from build123d import *

# Parameters (mm, degrees)
SKETCH1_W           = 13
SKETCH1_H           = 18
BOSS_EXTRUDE1_DEPTH = 3.2
SKETCH2_W           = 15
SKETCH2_H           = 20
BOSS_EXTRUDE2_DEPTH = 1
SKETCH3_R           = 1.5
CUT_EXTRUDE1_DEPTH  = 14.18673576
FILLET1_R           = 0.2
FILLET2_R           = 1


with BuildPart() as part:
    # Sketch1 → Boss-Extrude1 (new body)
    with BuildSketch(Plane(origin=(0, 0, 0), x_dir=(1, 0, 0), z_dir=(0, 1, 0))):
        Rectangle(SKETCH1_W, SKETCH1_H)
    extrude(amount=BOSS_EXTRUDE1_DEPTH)

    # Sketch2 → Boss-Extrude2 (add)
    with BuildSketch(Plane(origin=(0, 3.2, 0), x_dir=(1, 0, 0), z_dir=(0, 1, 0))):
        Rectangle(SKETCH2_W, SKETCH2_H)
    extrude(amount=BOSS_EXTRUDE2_DEPTH)

    # Sketch3 → Cut-Extrude1 (cut, through all)
    with BuildSketch(Plane.XZ):
        with Locations(Location((0, 3, 0), (0, 0, 270))):
            Circle(SKETCH3_R)
        with Locations(Location((0, -3, 0), (0, 0, 270))):
            Circle(SKETCH3_R)
        Polygon((4.8, -5.5), (-1.3, -5.5), (-1.3, -5.9), (5.5, -5.9), (5.5, 8), (4.8, 8), align=None)
        Polygon((2.5, 7.85), (2.5, -4.3), (3.6, -4.3), (3.6, 8), (-5.5, 8), (-5.5, 7.6), (1.5, 7.6), (1.5, 7.85), align=None)
        Polygon((-2.5, -7.1), (-2.5, 4.3), (-3.9, 4.3), (-3.9, -8), (5.5, -8), (5.5, -7.1), align=None)
        Polygon((-5.35, 5.5), (1.3, 5.5), (1.3, 6.4), (-5.5, 6.4), (-5.5, -8), (-5.1, -8), (-5.1, 4.3), (-5.35, 4.3), align=None)
    extrude(amount=-CUT_EXTRUDE1_DEPTH, mode=Mode.SUBTRACT)

    # Fillet1
    fillet1_edges = [part.edges().sort_by_distance(p)[0] for p in [
        (-5.1, 2.1, -8),
        (-3.9, 2.1, -8),
        (-5.5, 2.1, 6.4),
        (-5.5, 2.1, 7.6),
        (4.8, 2.1, 8),
        (3.6, 2.1, 8),
        (-3.9, 2.1, 4.3),
        (-2.5, 2.1, 4.3),
        (1.3, 2.1, 5.5),
        (1.3, 2.1, 6.4),
        (5.5, 2.1, -7.1),
        (5.5, 2.1, -5.9),
        (-1.3, 2.1, -5.9),
        (-1.3, 2.1, -5.5),
        (3.6, 2.1, -4.3),
        (2.5, 2.1, -4.3),
    ]]
    fillet(fillet1_edges, radius=FILLET1_R - 0.0001)  # a hair under: the kernel refuses the full size

    # Fillet2
    fillet2_edges = [part.edges().sort_by_distance(p)[0] for p in [
        (6.5, 1.6, 9),
        (-6.5, 1.6, 9),
        (-6.5, 1.6, -9),
        (6.5, 1.6, -9),
    ]]
    fillet(fillet2_edges, radius=FILLET2_R)


with BuildPart() as body_2:
    # Mirror1: mirrored copy
    add(part.part.mirror(Plane(origin=(-7.5, 4.2, -10), x_dir=(0, 0, 1), z_dir=(1, 0, 0))))


solid = body_2.part
CAD build for the part. Positions are in the model's coordinates, mm. A direction names the side the tool comes from. Give positions to 0.01 mm unless a question says otherwise; leave off trailing zeros. Loops run counter-clockwise (first coordinate to the right, second up) from the corner with the lowest first, then second, coordinate; pieces in that order, holes last. Notation, with made-up numbers: M -5,62.5 L -1,62.5 A13 cw -1,77.5 Z; hole C -30,-3 d5. An arc over 180 degrees is marked long. Answer in a Markdown table with one row per item. Add a question column.
Item 1: Mould opens along X. For faces 1 (the face through (-8.785, 1.622, 8.699)), 2 (the face through (-15, 4.2, 0)), 3 (the face through (-17, 2, 7.85)), 4 (the face through (-22.5, 4, 0)) say: +X half, -X half, draft (parallel to the pull), parting line (faces both ways), or undercut.
Item 2: Band-saw the part on A-A on z = 3. Give the cut face in (x, y), then the cut area to 3 significant figures.
Item 3: Tool access for faces 5 (the face through (-15, 2, -9)), 6 (the face through (-17, 2, -5.5)), 7 (the face through (-8.5, 2, 0)): list every direction of +Z, -Z, +X, -X, +Y, -Y with a clear straight run to the whole face (end or side of a thin tool).
Item 4: Drop flat-ended pins along their axis: P1, Ø1.3, axis at y = 2, z = 0.5, coming from the +X side; P2, Ø1.3, axis at y = 1.5, z = -3, coming from the -X side; P3, Ø2.5, axis at y = 2, z = 2.5, coming from the -X side; P4, Ø2, axis at x = -14, y = 2, coming from the +Z side. Give the stop position or say it passes through.
Item 5: Band-saw the part on B-B on x = -15. Give the number of separate pieces and of enclosed holes in the cut face, then the cut area to 3 significant figures.
Item 6: Probe probe 1 along Z at (x, y) = (-10.5, 1.7); probe 2 along Z at (x, y) = (-19.5, 1.45); probe 3 along X at (y, z) = (2.5, 5.75). List the from-to ranges inside material, lowest first.
Item 7: Band-saw the part on D-D on z = -2.25. Give the cut face in (x, y).
Reply:
| question | item | result |
|---|---|---|
| 1 | face 1 | +X half |
| 1 | face 2 | draft |
| 1 | face 3 | undercut |
| 1 | face 4 | -X half |
| 2 | outline | M -22.5,3.2 L -21.5,3.2 L -21.5,0 L -20.5,0 L -20.5,4.2 L -22.5,4.2 Z; M -19.8,0 L -18.6,0 L -18.6,4.2 L -19.8,4.2 Z; M -17.5,0 L -16.5,0 L -16.5,4.2 L -17.5,4.2 Z; M -13.5,0 L -12.5,0 L -12.5,4.2 L -13.5,4.2 Z; M -11.1,0 L -9.9,0 L -9.9,4.2 L -11.1,4.2 Z; M -9.5,0 L -8.5,0 L -8.5,3.2 L -7.5,3.2 L -7.5,4.2 L -9.5,4.2 Z |
| 2 | area | 28.9 mm^2 |
| 3 | face 5 | -Z, +X, -X, -Y |
| 3 | face 6 | +Y, -Y |
| 3 | face 7 | +Z, -Z, +X, -Y |
| 4 | P1 | stops at x = -8.5 |
| 4 | P2 | stops at x = -21.5 |
| 4 | P3 | stops at x = -22.5 |
| 4 | P4 | stops at z = 9 |
| 5 | separate pieces | 7 |
| 5 | enclosed holes | 0 |
| 5 | area | 41.5 mm^2 |
| 6 | probe 1 | z = -9 to 5.5, 6.4 to 7.6, 8 to 9 |
| 6 | probe 2 | z = -9 to -8, -7.1 to -5.9, -5.5 to 9 |
| 6 | probe 3 | x = -21.5 to -20.5, -19.8 to -18.6, -17.5 to -16.3, -9.5 to -8.5 |
| 7 | outline | M -22.5,3.2 L -21.5,3.2 L -21.5,0 L -20.5,0 L -20.5,4.2 L -22.5,4.2 Z; M -19.8,0 L -18.6,0 L -18.6,4.2 L -19.8,4.2 Z; M -17.5,0 L -16.3,0 L -16.3,4.2 L -17.5,4.2 Z; M -13.7,0 L -12.5,0 L -12.5,4.2 L -13.7,4.2 Z; M -11.1,0 L -9.9,0 L -9.9,4.2 L -11.1,4.2 Z; M -9.5,0 L -8.5,0 L -8.5,3.2 L -7.5,3.2 L -7.5,4.2 L -9.5,4.2 Z |
